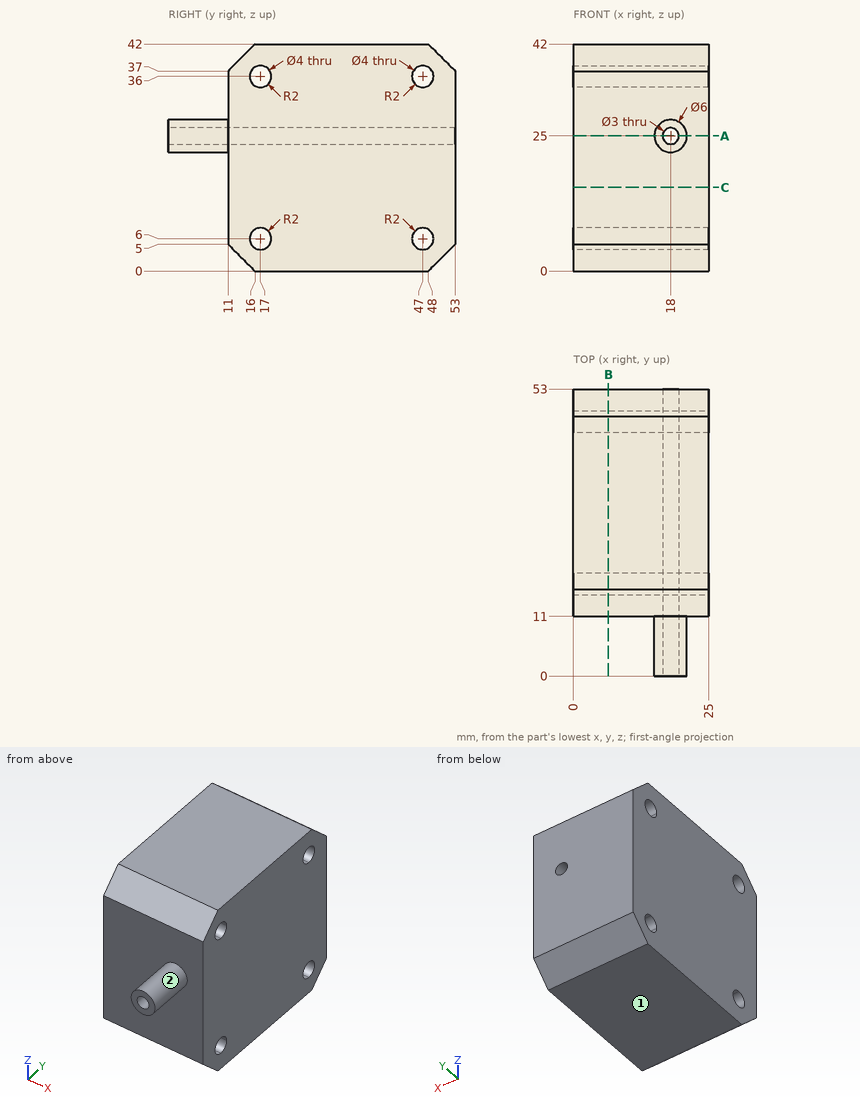
The figure shows three views and two pictorial views of one solid part (mm, origin at its lowest corner). Answer the questions. A direction names the side the tool comes from. Round coordinates to 2 decimals unless told otherwise and drop trailing zeros. Order: outer loops, then holes, each group sorted by start corner. A loop starts at its lowest first (then second) coordinate and runs counter-clockwise, first axis right, second up. Notation, with made-up numbers: (54.25, 84.25) - (100.25, 84.25) arc R22 cw to (100.25, 100.25) - close; hole circle Ø1 at (-30.5, 27). An arc over 180 degrees is marked (long way). Write item = value, one per line. Start each with the question number.
1) Section B-B, the plane x = 6.5 is taken. Write down the section's boundary in (y, z), plus the area to 3 significant figures.
2) Section A-A, the plane z = 25 is taken. Write down the section's boundary in (x, y).
3) Section C-C, the plane z = 15.5 is taken. Write down the section's boundary in (x, y), plus the area to 3 significant figures.
4) Given pin 1 (2 mm diameter, centred on x = 19.5, z = 35.5, fed in from -Y); pin 2 (10 mm diameter, centred on x = 20, y = 8, fed in from +Z); pin 3 (2 mm diameter, centred on x = 21, y = 13, fed in from +Z), each flat-ended and moving along its own axis, determine where each tip first touches the part or whether it passes through.
5) Straight lines are drawn through the part: L1, parallel to Y at x = 7.5, z = 36; L2, parallel to Z at x = 15.5, y = 17; L3, parallel to X at y = 15, z = 25. For each, find the intervals that lie inside material, in ascending order.
6) For the marked faces 1 and 2, determine the directions among +Z, -Z, +X, -X, +Y, -Y from which every point of the face is accessible in a straight line to the end or side of a thin tool.
Results list:
q1.outline = (11, 5) - (16, 0) - (48, 0) - (53, 5) - (53, 37) - (48, 42) - (16, 42) - (11, 37) - close; hole circle Ø4 at (17, 6); hole circle Ø4 at (17, 36); hole circle Ø4 at (47, 6); hole circle Ø4 at (47, 36)
q1.area = 1,660 mm^2
q2.outline = (0, 11) - (15, 11) - (15, 0) - (16.5, 0) - (16.5, 53) - (0, 53) - close; (19.5, 0) - (21, 0) - (21, 11) - (25, 11) - (25, 53) - (19.5, 53) - close
q3.outline = (0, 11) - (25, 11) - (25, 53) - (0, 53) - close
q3.area = 1,050 mm^2
q4.pin_1 = 11
q4.pin_2 = 39
q4.pin_3 = 40
q5.L1 = 11 to 15, 19 to 45, 49 to 53
q5.L2 = 0 to 4, 8 to 34, 38 to 42
q5.L3 = 0 to 16.5, 19.5 to 25
q6.face_1 = -Z, +X, -X, +Y, -Y
q6.face_2 = -Y
